```python
from build123d import *

# Parameters (mm, degrees)
F1_ANGLE_BACK = 22.5
F1_ANGLE      = 45
F2_R          = 1.125
F3_DEPTH      = 24
F5_DEPTH      = 10
F6_R          = 10
F7_R          = 5
F8_R          = 7


with BuildPart() as f1:
    # F0 (on Right) → F1 (revolve)
    with BuildSketch(Plane.YZ, mode=Mode.PRIVATE) as f1_sk:
        Polygon((10, 10), (10, -10), (-10, -10), (-10, 10), (-12, 10), (-12, -12), (12, -12), (12, 10), align=None)
    revolve(f1_sk.sketch.rotate(Axis((0, -36.9127653539, -112), (0, -1, 0)), -F1_ANGLE_BACK), axis=Axis((0, -36.9127653539, -112), (0, -1, 0)), revolution_arc=F1_ANGLE)

    # F2 (on face) → F3 (join)
    with BuildSketch(Plane.XZ.offset(12)):
        with BuildLine():
            Line((6.3674504599, 9.8337210079), (1.178053683, 13.6162269395))
            ThreePointArc((1.178053683, 13.6162269395), (0, 14), (-1.178053683, 13.6162269395))
            Line((-1.178053683, 13.6162269395), (-6.3674504599, 9.8337210079))
            ThreePointArc((-6.3674504599, 9.8337210079), (0, 10), (6.3674504599, 9.8337210079))
        make_face()
        with Locations((0, 12)):
            Circle(F2_R, mode=Mode.SUBTRACT)
    extrude(amount=-F3_DEPTH)

    # F4 (on Right) → F5 (cut, symmetric)
    with BuildSketch(Plane.YZ):
        Polygon((-10, 0), (0, 0), (10, 0), (10, 19.6699723601), (-10, 19.6699723601), align=None)
    extrude(amount=F5_DEPTH, both=True, mode=Mode.SUBTRACT)

    # F6
    f6_edges = [f1.edges().sort_by_distance(p)[0] for p in [
        (-46.687379, 11, 0.713303),
        (-46.687379, -11, 0.713303),
        (46.687379, -11, 0.713303),
        (46.687379, 11, 0.713303),
    ]]
    fillet(f6_edges, radius=F6_R)

    # F7
    f7_edges = [f1.edges().sort_by_distance(p)[0] for p in [
        (0, 10, -10),
        (0, -10, -10),
    ]]
    fillet(f7_edges, radius=F7_R)

    # F8
    f8_edges = [f1.edges().sort_by_distance(p)[0] for p in [
        (0, 12, -12),
        (0, -12, -12),
    ]]
    fillet(f8_edges, radius=F8_R)


solid = f1.part
```
Can you work these out from the model? Positions are in its coordinate system, mm. A direction names the side the tool comes from. Round coordinates to 2 decimals unless told otherwise and drop trailing zeros. Loops run counter-clockwise (first coordinate to the right, second up) from the corner with the lowest first, then second, coordinate; pieces in that order, holes last. Notation, with made-up numbers: (84.5, 1.25) -> (109.5, 1.25) arc R21 cw to (109.5, 10.25) -> close; hole circle Ø4 at (-18.5, 48). An arc over 180 degrees is marked (long way). Answer in a Markdown table with one row per item.
Item 1: If I drill on probe 1 along Y at (x, z) = (25, -5.5); probe 2 along Y at (x, z) = (-29, -10); probe 3 along Z at (x, y) = (-8, -8.5), over which ranges is the centre line in solid material (lowest first)?
Answer block:
| item | result |
|---|---|
| probe 1 | -12 to -10, 10 to 12 |
| probe 2 | -11.93 to -9.91, 9.91 to 11.93 |
| probe 3 | -11.38 to -8.88 |
Item 2: On a 3-axis mill with a long thin cutter (end or side, diameter ignored), from which of +Z, -Z, +X, -X, +Y, -Y can I reach the whole of each face in a straight line? I mean faces 1 (the flat face through (1, -10, 1)), 2 (the cylindrical face through (42.558, 10.986, -0.982)). Say none if no direction works.
Answer block:
| item | result |
|---|---|
| face 1 | +Z |
| face 2 | +X, +Y, -Y |
Item 3: Suppose I cut it at C-C, the plane z = -2. List the corners of the cut face in (x, y) for me, plus the area to 3 significant figures.
Answer block:
| item | result |
|---|---|
| outline | (-42.95, -12) -> (42.95, -12) -> (42.95, -10) -> (-42.95, -10) -> close; (-42.95, 10) -> (42.95, 10) -> (42.95, 12) -> (-42.95, 12) -> close |
| area | 344 mm² |
Item 4: Suppose I cut it at D-D, the plane y = 4. List the corners of the cut face in (x, z) for me.
Answer block:
| item | result |
|---|---|
| outline | (-39.03, -17.76) -> (-38.27, -19.61) arc R100 cw to (38.27, -19.61) -> (39.03, -17.76) arc R102 ccw to start |
Item 5: Suppose I cut it at A-A, the plane x = 0. List the corners of the cut face in (y, z) for me (3 decimals).
Answer block:
| item | result |
|---|---|
| outline | (-12, -5) arc R7 ccw to (-5, -12) -> (5, -12) arc R7 ccw to (12, -5) -> (12, 10.875) -> (10, 10.875) -> (10, -5) arc R5 cw to (5, -10) -> (-5, -10) arc R5 cw to (-10, -5) -> (-10, 10.875) -> (-12, 10.875) -> close; (-12, 13.125) -> (-10, 13.125) -> (-10, 14) -> (-12, 14) -> close; (10, 13.125) -> (12, 13.125) -> (12, 14) -> (10, 14) -> close |
Item 6: We'd pull the mould along Z, two halves only. Please class faces 3 (the cylindrical face through (-21.361, -11.014, 8.115)), 4 (the flat face through (-1, 12, 1)), 5 (the cylindrical face through (-0.24, -11.01, 10.9)): released by +Z, released by -Z, zero draft, split by the parting line, or undercut.
Answer block:
| item | result |
|---|---|
| face 3 | released by +Z |
| face 4 | zero draft |
| face 5 | undercut |
Item 7: Will these pins go through, and if not, where does the flat tip stop? P1, Ø1.3, axis at x = 0, z = 12, coming from the +Y side; P2, Ø6, axis at x = -13.5, z = -13.5, coming from the -Y side; P3, Ø5, axis at x = 26, y = 6, coming from the +Z side; P4, Ø2, axis at x = 8, y = -7.5, coming from the -Z side.
Answer block:
| item | result |
|---|---|
| P1 | through |
| P2 | y = -10.29 |
| P3 | z = -11.81 |
| P4 | z = -12.17 |
Item 8: Suppose I cut it at B-B, the plane z = 12. List the corners of the cut face in (x, y) for me (3 decimals), plus the area to 3 significant figures.
Answer block:
| item | result |
|---|---|
| outline | (-3.395, -12) -> (-1.125, -12) -> (-1.125, -10) -> (-3.395, -10) -> close; (-3.395, 10) -> (-1.125, 10) -> (-1.125, 12) -> (-3.395, 12) -> close; (1.125, -12) -> (3.395, -12) -> (3.395, -10) -> (1.125, -10) -> close; (1.125, 10) -> (3.395, 10) -> (3.395, 12) -> (1.125, 12) -> close |
| area | 18.2 mm² |
